CAD build for the part. Positions are in the model's coordinates, mm. Coordinates: 2 decimals unless noted, no trailing zeros. Loops run counter-clockwise (first coordinate to the right, second up) from the corner with the lowest first, then second, coordinate; pieces in that order, holes last. Notation, with made-up numbers: (27, 14.25) -> (48, 14.25) arc R29 ccw to (48, 35.25) -> close; hole circle Ø3 at (37.25, 30.5). An arc over 180 degrees is marked (long way). Answer as a JSON object with one key per item and string values. Group by question number.
from build123d import *

# Parameters (mm, degrees)
SKETCH_1_W                  = 73
SKETCH_1_H                  = 53
EXTRUDE_1_DEPTH             = 1.5
FILLET_1_R                  = 2
SKETCH_2_R                  = 1.6
CUT_EXTRUDE_1_DEPTH         = 46.130366717
PATTERN_LINEAR_1_COUNT      = 2
PATTERN_LINEAR_1_PITCH      = 60
PATTERN_LINEAR_1_COUNT_DIR2 = 2
PATTERN_LINEAR_1_PITCH_DIR2 = 40


with BuildPart() as part:
    # 草图1 → 凸台-拉伸1 (new body)
    with BuildSketch(Plane(origin=(0, 0, 0), x_dir=(1, 0, 0), z_dir=(0, 1, 0))):
        Rectangle(SKETCH_1_W, SKETCH_1_H)
    extrude(amount=EXTRUDE_1_DEPTH)

    # 圆角1
    fillet_1_edges = [part.edges().sort_by_distance(p)[0] for p in [
        (-36.5, 0.75, -26.5),
        (36.5, 0.75, -26.5),
        (36.5, 0.75, 26.5),
        (-36.5, 0.75, 26.5),
    ]]
    fillet(fillet_1_edges, radius=FILLET_1_R)

    # 草图2 → 切除-拉伸1 (cut, through all)
    with BuildSketch(Plane(origin=(0, 1.5, 0), x_dir=(1, 0, 0), z_dir=(0, 1, 0))):
        with Locations(Location((-30, 20, 0), (0, 0, 270))):
            Circle(SKETCH_2_R)
    cut_extrude_1 = extrude(amount=-CUT_EXTRUDE_1_DEPTH, mode=Mode.SUBTRACT)

    # 阵列(线性)1: Cut-Extrude 1 2 × 2
    with Locations(*[(i * PATTERN_LINEAR_1_PITCH, 0, j * PATTERN_LINEAR_1_PITCH_DIR2) for i in range(PATTERN_LINEAR_1_COUNT) for j in range(PATTERN_LINEAR_1_COUNT_DIR2) if (i, j) != (0, 0)]):
        add(cut_extrude_1, mode=Mode.SUBTRACT)


solid = part.part
Item 1: Flat gauge pin, fed straight in: P1, Ø3, axis at x = -30, z = -20, coming from the -Y side. Where does the tip first touch, or does it go through?
Item 2: Drill centre lines: L1, parallel to X at y = 0.8, z = -20; L2, parallel to Z at x = -30.5, y = 0.85. Where is each one in solid material? Low to high.
Item 3: Pull direction X, two halves, no side cores. Call faces 1 (the cylindrical face through (-35.93, 0.76, -25.9)), 2 (the flat face through (-1, 0, 0)), 3 (the cylindrical face through (31.08, 0.76, 18.82)): +X half, -X half, draft (parallel to the pull), parting line (faces both ways), or undercut.
Item 4: Band-saw the part on B-B, the plane z = 20. List the corners of the cut face in (x, y), and give its area (3 significant figures).
Item 5: Band-saw the part on A-A, the plane x = -30. List the corners of the cut face in (y, z), and give its area (3 significant figures).
Reply:
{
 "1": {"P1": "through"},
 "2": {"L1": "-36.5 to -31.6, -28.4 to 28.4, 31.6 to 36.5", "L2": "-26.5 to -21.52, -18.48 to 18.48, 21.52 to 26.5"},
 "3": {"face 1": "-X half", "face 2": "draft", "face 3": "undercut"},
 "4": {"outline": "(-36.5, 0) -> (-31.6, 0) -> (-31.6, 1.5) -> (-36.5, 1.5) -> close; (-28.4, 0) -> (28.4, 0) -> (28.4, 1.5) -> (-28.4, 1.5) -> close; (31.6, 0) -> (36.5, 0) -> (36.5, 1.5) -> (31.6, 1.5) -> close", "area": "99.9 mm²"},
 "5": {"outline": "(0, -26.5) -> (1.5, -26.5) -> (1.5, -21.6) -> (0, -21.6) -> close; (0, -18.4) -> (1.5, -18.4) -> (1.5, 18.4) -> (0, 18.4) -> close; (0, 21.6) -> (1.5, 21.6) -> (1.5, 26.5) -> (0, 26.5) -> close", "area": "69.9 mm²"}
}
